Geometry check sheet. Reference: the model listing, model coordinates, mm. Face numbers are marked on the shaded views. A direction names the side the tool comes from. Round coordinates to 2 decimals unless told otherwise and drop trailing zeros. Loops run counter-clockwise (first coordinate to the right, second up) from the corner with the lowest first, then second, coordinate; pieces in that order, holes last. Notation, with made-up numbers: (4.25, -6.75) -> (23.25, -6.75) arc R29 cw to (23.25, 19.25) -> close; hole circle Ø2 at (26.5, -17.5). An arc over 180 degrees is marked (long way). Use a Markdown table: item, result. Add a question column.
Q1. Sectioned sample at A-A, the plane x = 0. Enter the section's corners in (y, z).
Q2. Gauge pin test, flat ends, axial feed: P1, Ø2, axis at x = -7, y = 3, coming from the -Z side; P2, Ø1.5, axis at y = 3.5, z = 8, coming from the +X side; P3, Ø1.5, axis at y = 6.5, z = -4.5, coming from the -X side. Record the tip position at first contact, or that the pin passes through.
Q3. Sectioned sample at B-B, the plane z = 0. Enter the section's corners in (x, y).
Q4. Release check for a two-part mould opening along Z. For the marked faces 3 and 4 record: released by +Z, released by -Z, zero draft, split by the parting line, or undercut.
Q5. Sectioned sample at C-C, the plane y = 3. Enter the section's corners in (x, z).
Q6. Set-up check for the marked faces 1 and 2: record each of +Z, -Z, +X, -X, +Y, -Y from which the full face is reachable in a straight line by a thin tool's end or side.
Q7. Material ranges on L1, parallel to Y at x = -10.5, z = -1; L2, parallel to X at y = 1.85, z = 0; L3, parallel to Z at x = -8, y = 0.75, recorded low to high.
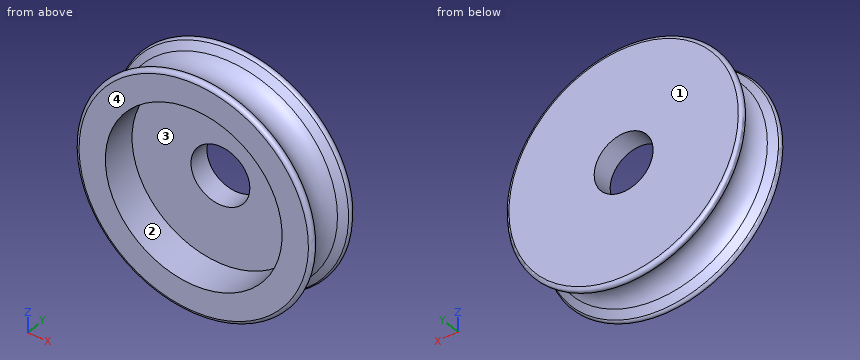
```python
from build123d import *

# Parameters (mm, degrees)
SKETCH_1_R          = 17
EXTRUDE_1_DEPTH     = 8
SKETCH_2_R          = 12
CUT_EXTRUDE_2_DEPTH = 5
FILLET_1_R          = 0.5
SKETCH_5_R          = 4
CUT_EXTRUDE_3_DEPTH = 25.099505092


with BuildPart() as part:
    # Эскиз1 → Вытянуть1 (new body)
    with BuildSketch(Plane(origin=(0, 0, 0), x_dir=(1, 0, 0), z_dir=(0, 1, 0))):
        with Locations(Location((0, 0, 0), (0, 0, 270))):
            Circle(SKETCH_1_R)
    extrude(amount=EXTRUDE_1_DEPTH)

    # Эскиз2 → Вытянуть2 (cut)
    with BuildSketch(Plane.XZ):
        with Locations(Location((0, 0, 0), (0, 0, 270))):
            Circle(SKETCH_2_R)
    extrude(amount=-CUT_EXTRUDE_2_DEPTH, mode=Mode.SUBTRACT)

    # Эскиз4 → Вырез-Повернуть1 (revolve, cut)
    with BuildSketch(Plane(origin=(0, 0, 0), x_dir=(0, 0, -1), z_dir=(1, 0, 0))):
        with BuildLine():
            Line((17, 8), (14.928258035, 6.342606428))
            ThreePointArc((14.928258035, 6.342606428), (13.802343178, 4), (14.928258035, 1.657393572))
            Line((14.928258035, 1.657393572), (17, 0))
            Line((17, 0), (17, 8))
        make_face()
    revolve(axis=Axis((0, 11, 0), (0, 1, 0)), mode=Mode.SUBTRACT)

    # Скругление1
    fillet_1_edges = [part.edges().sort_by_distance(p)[0] for p in [
        (0, 8, 17),
        (0, 0, 17),
    ]]
    fillet(fillet_1_edges, radius=FILLET_1_R)

    # Эскиз5 → Вытянуть3 (cut, through all)
    with BuildSketch(Plane(origin=(0, 8, 0), x_dir=(1, 0, 0), z_dir=(0, 1, 0))):
        with Locations(Location((0, 0, 0), (0, 0, 270))):
            Circle(SKETCH_5_R)
    extrude(amount=-CUT_EXTRUDE_3_DEPTH, mode=Mode.SUBTRACT)


solid = part.part
```
Values:
| question | item | result |
|---|---|---|
| 1 | outline | (0, -15.57) arc R0.5 ccw to (0.89, -15.89) -> (1.66, -14.93) arc R3 cw to (6.34, -14.93) -> (7.11, -15.89) arc R0.5 ccw to (8, -15.57) -> (8, -4) -> (5, -4) -> (5, -12) -> (0, -12) -> close; (0, 12) -> (5, 12) -> (5, 4) -> (8, 4) -> (8, 15.57) arc R0.5 ccw to (7.11, 15.89) -> (6.34, 14.93) arc R3 cw to (1.66, 14.93) -> (0.89, 15.89) arc R0.5 ccw to (0, 15.57) -> close |
| 2 | P1 | z = -12.91 |
| 2 | P2 | x = 11.84 |
| 2 | P3 | x = -15.4 |
| 3 | outline | (-15.89, 0.89) arc R0.5 ccw to (-15.57, 0) -> (-12, 0) -> (-12, 5) -> (-4, 5) -> (-4, 8) -> (-15.57, 8) arc R0.5 ccw to (-15.89, 7.11) -> (-14.93, 6.34) arc R3 cw to (-14.93, 1.66) -> close; (4, 5) -> (12, 5) -> (12, 0) -> (15.57, 0) arc R0.5 ccw to (15.89, 0.89) -> (14.93, 1.66) arc R3 cw to (14.93, 6.34) -> (15.89, 7.11) arc R0.5 ccw to (15.57, 8) -> (4, 8) -> close |
| 4 | face 3 | undercut |
| 4 | face 4 | zero draft |
| 5 | outline | circle Ø27.95 at (0, 0); hole circle Ø24 at (0, 0) |
| 6 | face 1 | +Z, -Z, +X, -X, +Y |
| 6 | face 2 | -Y |
| 7 | L1 | 5 to 8 |
| 7 | L2 | -14.71 to -12, 12 to 14.71 |
| 7 | L3 | -13.87 to -8.94, 8.94 to 13.87 |
